Read the model definition and answer for the solid it produces. Units are mm, in the model's axes. A direction names the side the tool comes from. Round coordinates to 2 decimals unless told otherwise and drop trailing zeros. Order: outer loops, then holes, each group sorted by start corner. A loop starts at its lowest first (then second) coordinate and runs counter-clockwise, first axis right, second up. Notation, with made-up numbers: (47, 23.5) -> (60, 23.5) arc R16 cw to (60, 45.5) -> close; hole circle Ø9 at (-14.5, -14.5). An arc over 180 degrees is marked (long way). Use a Markdown table: item, result. Add a question column.
1. For faces 1 (the face through (-0.32, -8.85, 2.58)), 2 (the face through (1, -1, 15.24)), determine the directions among +Z, -Z, +X, -X, +Y, -Y from which every point of the face is accessible in a straight line to the end or side of a thin tool.
2. Given pin 1 (2 mm diameter, centred on x = -25, y = -22.5, fed in from +Z); pin 2 (8 mm diameter, centred on y = 50.5, z = 6.5, fed in from +X); pin 3 (3 mm diameter, centred on y = -17, z = 4.5, fed in from -X); pin 4 (15 mm diameter, centred on x = 44.73, y = 44.73, fed in from +Z), each flat-ended and moving along its own axis, determine where each tip first touches the part or whether it passes through.
3. Section B-B, the plane z = 3 is taken. Give the vertices of the cut face in (x, y).
4. Section D-D, the plane y = 0 is taken. Give the vertices of the cut face in (x, z), then the cut area to 3 significant figures.
5. Consider L1, parallel to X at y = 39, z = 3; L2, parallel to Z at x = 54.5, y = 52.5; L3, parallel to X at y = 51.5, z = 3.25. Determine where each line is inside the solid, lowest interval first. Write a range as [from, to].
6. Section C-C, the plane x = 0 is taken. Give the vertices of the cut face in (y, z).
7. Section A-A, the plane y = 49 is taken. Give the vertices of the cut face in (x, z).
8. The mould has two halves that part along Y. Classify faces 3 (the face through (17.51, 3.59, 10.09)), 4 (the face through (-1, 14, 0)), 5 (the face through (53.657, 47.542, 2.504)): +Y half, -Y half, draft (parallel to the pull), parting line (faces both ways), or undercut.
```python
from build123d import *

# Parameters (mm, degrees)
SKETCH1_R           = 8.332963545
SKETCH1_R_2         = 9.35840883
BOSS_EXTRUDE2_DEPTH = 5.08
SKETCH2_R           = 16.987426911
BOSS_EXTRUDE3_DEPTH = 10.16
SKETCH2_3_R         = 7.512157001
CUT_EXTRUDE1_DEPTH  = 10.16
SKETCH2_4_R         = 16.987426911
SKETCH2_4_R_2       = 7.512157001
BOSS_EXTRUDE4_DEPTH = 10.16


with BuildPart() as part:
    # Sketch1 → Boss-Extrude2 (new body)
    with BuildSketch(Plane.XY):
        with BuildLine():
            ThreePointArc((-40.42750083, 19.142632152), (0.054998173, -44.730528326), (40.380305232, 19.241988943))
            ThreePointArc((40.380305232, 19.241988943), (63.014326775, 63.014326775), (19.241988943, 40.380305232))
            ThreePointArc((19.241988943, 40.380305232), (0.054998173, 44.730528326), (-19.142632152, 40.42750083))
            ThreePointArc((-19.142632152, 40.42750083), (-63.078021056, 63.078021056), (-40.42750083, 19.142632152))
        make_face()
        with Locations((-44.730562137, 44.730562137)):
            Circle(SKETCH1_R, mode=Mode.SUBTRACT)
        with Locations((44.730562137, 44.730562137)):
            Circle(SKETCH1_R_2, mode=Mode.SUBTRACT)
    extrude(amount=BOSS_EXTRUDE2_DEPTH)

    # Sketch2 → Boss-Extrude3 (add)
    with BuildSketch(Plane.XY.offset(5.08)):
        with Locations((1.305897397, -1.51434167)):
            Circle(SKETCH2_R)
    extrude(amount=BOSS_EXTRUDE3_DEPTH)

    # Sketch2<3> → Cut-Extrude1 (cut)
    with BuildSketch(Plane.XY.offset(5.08)):
        with Locations((1.305897397, -1.51434167)):
            Circle(SKETCH2_3_R)
    extrude(amount=-CUT_EXTRUDE1_DEPTH, mode=Mode.SUBTRACT)

    # Sketch2<4> → Boss-Extrude4 (add, through all)
    with BuildSketch(Plane.XY.offset(5.08)):
        with Locations((1.305897397, -1.51434167)):
            Circle(SKETCH2_4_R)
        with Locations((1.305897397, -1.51434167)):
            Circle(SKETCH2_4_R_2, mode=Mode.SUBTRACT)
    extrude(amount=BOSS_EXTRUDE4_DEPTH)


solid = part.part
```
Verdict:
| question | item | result |
|---|---|---|
| 1 | face 1 | -Z |
| 1 | face 2 | +Z, +X, -X, +Y, -Y |
| 2 | pin 1 | stops at z = 5.08 |
| 2 | pin 2 | stops at x = 70.51 |
| 2 | pin 3 | stops at x = -41.96 |
| 2 | pin 4 | passes through |
| 3 | outline | (-40.43, 19.14) arc R44.73 ccw (long way) to (40.38, 19.24) arc R25.86 ccw (long way) to (19.24, 40.38) arc R44.73 ccw to (-19.14, 40.43) arc R25.95 ccw (long way) to start; hole circle Ø16.67 at (-44.73, 44.73); hole circle Ø15.02 at (1.31, -1.51); hole circle Ø18.72 at (44.73, 44.73) |
| 4 | outline | (-44.73, 0) -> (-6.05, 0) -> (-6.05, 5.08) -> (8.66, 5.08) -> (8.66, 0) -> (44.73, 0) -> (44.73, 5.08) -> (18.23, 5.08) -> (18.23, 15.24) -> (-15.61, 15.24) -> (-15.61, 5.08) -> (-44.73, 5.08) -> close |
| 4 | area | 724 mm2 |
| 5 | L1 | x = [-70.04, -50.78], [-38.68, 37.33], [52.13, 69.94] |
| 5 | L2 | z = [0, 5.08] |
| 5 | L3 | x = [-69.78, -49.59], [-39.87, -19.68], [19.78, 38.27], [51.19, 69.69] |
| 6 | outline | (-44.73, 0) -> (-8.91, 0) -> (-8.91, 5.08) -> (5.88, 5.08) -> (5.88, 0) -> (44.73, 0) -> (44.73, 5.08) -> (15.42, 5.08) -> (15.42, 15.24) -> (-18.45, 15.24) -> (-18.45, 5.08) -> (-44.73, 5.08) -> close |
| 7 | outline | (-70.32, 0) -> (-51.89, 0) -> (-51.89, 5.08) -> (-70.32, 5.08) -> close; (-37.57, 0) -> (-19.14, 0) -> (-19.14, 5.08) -> (-37.57, 5.08) -> close; (19.23, 0) -> (36.4, 0) -> (36.4, 5.08) -> (19.23, 5.08) -> close; (53.06, 0) -> (70.23, 0) -> (70.23, 5.08) -> (53.06, 5.08) -> close |
| 8 | face 3 | parting line |
| 8 | face 4 | draft |
| 8 | face 5 | undercut |
